from build123d import *

# Parameters (mm, degrees)
F1_ANGLE = 180
F3_D     = 4.4
F6_R     = 2.2
F7_DEPTH = 19


with BuildPart() as f1:
    # F0 (on Front) → F1 (revolve)
    with BuildSketch(Plane.XZ):
        with BuildLine():
            Line((0, 24), (0, 13))
            Line((0, 13), (53, 13))
            Line((53, 13), (53, 17))
            Line((53, 17), (64, 17))
            Line((64, 17), (64, 13))
            Line((64, 13), (100, 13))
            Line((100, 13), (100, 0))
            Line((100, 0), (120, 0))
            add(Edge.make_bspline(
                [(10, 24), (14.5846361259, 24), (19.1911767131, 14.7073521681), (38.5291539725, 19.2623560501), (77.4336550451, 22.1476524592), (112.1829708833, 14.2248736546), (119.6026350157, 7.3835916313), (120, 0)],
                knots=[0, 0, 0, 0, 0.1438984957, 0.3179448336, 0.5884486431, 0.835948418, 1, 1, 1, 1], degree=3))
            Line((10, 24), (0, 24))
        make_face()
    revolve(axis=Axis((50, 0, 0), (1, 0, 0)), revolution_arc=F1_ANGLE)

    # F3 (through all)
    with Locations(Plane(origin=(0, 0, 0), x_dir=(1, 0, 0), z_dir=(0, 1, 0))):
        with Locations((6, -17), (6, 17), (106, 0)):
            Hole(F3_D / 2)

    # F6 (on plane+point) → F7 (cut)
    with BuildSketch(Plane.XZ.offset(24)):
        Polygon((9.6, 14.9215390309), (9.6, 19.0784609691), (6, 21.1569219382), (2.4, 19.0784609691), (2.4, 14.9215390309), (6, 12.8430780618), align=None)
        with Locations((6, 17)):
            Circle(F6_R, mode=Mode.SUBTRACT)
        Polygon((9.6, -19.0784609691), (9.6, -14.9215390309), (6, -12.8430780618), (2.4, -14.9215390309), (2.4, -19.0784609691), (6, -21.1569219382), align=None)
        with Locations((6, -17)):
            Circle(F6_R, mode=Mode.SUBTRACT)
        Polygon((109.6, -2.0784609691), (109.6, 2.0784609691), (106, 4.1569219382), (102.4, 2.0784609691), (102.4, -2.0784609691), (106, -4.1569219382), align=None)
        with Locations((106, 0)):
            Circle(F6_R, mode=Mode.SUBTRACT)
    extrude(amount=-F7_DEPTH, mode=Mode.SUBTRACT)


solid = f1.part
Read the model definition and answer for the solid it produces. Units are mm, in the model's axes. A direction names the side the tool comes from. Give positions to 0.01 mm unless a question says otherwise; leave off trailing zeros. Use CSV: the item, a comma, the result in double quotes. Start each with the question number.
Item 1: The part is cut by section A-A, the plane y = -8.5. Count the separate pieces of the cut face and the enclosed holes in it, and give its area (3 significant figures).
Item 2: Consider line 1 (Z direction, x = 6, y = -3.1); line 2 (Z direction, x = 6, y = -3.9); line 3 (X direction, y = -3.25, z = 0.5). Determine where each line is inside the solid, lowest interval first.
Item 3: The mould has two halves that part along X. Classify faces 4 (the flat face through (64.2, 0, 14.3)), 5 (the flat face through (0, -15, 0)), 6 (the flat face through (108, -10, -3)): pulls with the +X half, pulls with the -X half, needs draft (parallel to the pull), parting line crosses it, or undercut.
Item 4: For faces 1 (the cylindrical face through (59, -17, 0)), 2 (the flat face through (8, -9, 20)), 3 (the cylindrical face through (4.98, -2.53, 18.95)), determine the directions among +Z, -Z, +X, -X, +Y, -Y from which every point of the face is accessible in a straight line to the end or side of a thin tool.
Item 5: Flat-ended cylindrical pins translate along their axes: P1, Ø8, axis at x = 68.5, y = -16.5, coming from the -Z side; P2, Ø1.2, axis at y = -7, z = 0.5, coming from the -X side; P3, Ø8.5, axis at y = -4.5, z = 1.5, coming from the +X side. Find the tip coordinate at first contact, or state that the pin passes through.
Taken from the geometry:
1,separate pieces,"1"
1,enclosed holes,"3"
1,area,"1,700 mm2"
2,line 1,"-23.8 to -19.2, -14.8 to -12.62, 12.62 to 14.8, 19.2 to 23.8"
2,line 2,"-23.68 to -19.2, -14.8 to -12.4, 12.4 to 14.8, 19.2 to 23.68"
2,line 3,"100 to 103.86, 108.14 to 119.6"
3,face 4,"needs draft"
3,face 5,"pulls with the -X half"
3,face 6,"undercut"
4,face 1,"+Y"
4,face 2,"-Y"
4,face 3,"+Y, -Y"
5,P1,"z = -16.16"
5,P2,"x = 100"
5,P3,"x = 119.97"
